Work out the finished part from the listing and answer in its coordinate system (mm). A direction names the side the tool comes from. Give positions to 0.01 mm unless a question says otherwise; leave off trailing zeros. Order: outer loops, then holes, each group sorted by start corner. A loop starts at its lowest first (then second) coordinate and runs counter-clockwise, first axis right, second up. Notation, with made-up numbers: M 50,41.25 L 68,41.25 A22 cw 68,67.25 Z; hole C 2,-31.5 d7. An arc over 180 degrees is marked long. One line per item, written item: value.
from build123d import *

# Parameters (mm, degrees)
SKETCH_R     = 1.6
PAD_DEPTH    = 15
FILLET_R     = 5
SKETCH001_R  = 3
POCKET_DEPTH = 5


with BuildPart() as part:
    # Sketch → Pad (new body)
    with BuildSketch(Plane.XZ):
        with BuildLine():
            ThreePointArc((4.181539, 2.741301), (-4.970119, 0.54582), (3.486952, -3.583457))
            ThreePointArc((3.486952, -56.416543), (15, -30), (3.486952, -3.583457))
            ThreePointArc((3.486952, -56.416543), (-4.970119, -60.54582), (4.181539, -62.741301))
            Line((4.181539, -62.741301), (11.605736, -51.416543))
            ThreePointArc((11.605736, -51.416543), (18, -30), (11.605736, -8.583457))
            Line((4.181539, 2.741301), (11.605736, -8.583457))
        make_face()
        Circle(SKETCH_R, mode=Mode.SUBTRACT)
        with Locations((0, -60)):
            Circle(SKETCH_R, mode=Mode.SUBTRACT)
    extrude(amount=PAD_DEPTH)

    # Fillet
    fillet_edges = [part.edges().sort_by_distance(p)[0] for p in [
        (3.486952, -7.5, -3.583457),
        (3.486952, -7.5, -56.416543),
    ]]
    fillet(fillet_edges, radius=FILLET_R)

    # Sketch001 (on Face5 of Fillet) → Pocket (cut)
    with BuildSketch(Plane.XZ.offset(15)):
        Circle(SKETCH001_R)
        with Locations((0, -60)):
            Circle(SKETCH001_R)
    extrude(amount=-POCKET_DEPTH, mode=Mode.SUBTRACT)


solid = part.part
(1) Section B-B, the plane z = -60 is taken. Give the vertices of the cut face in (x, y).
Findings:
outline: M -5,-15 L -3,-15 L -3,-10 L -1.6,-10 L -1.6,0 L -5,0 Z; M 1.6,-10 L 3,-10 L 3,-15 L 5.98,-15 L 5.98,0 L 1.6,0 Z
(2) Section D-D, the plane z = -46 is taken. Give the vertices of the cut face in (x, y).
Findings:
outline: M 11.26,-15 L 14.57,-15 L 14.57,0 L 11.26,0 Z
(3) Section A-A, the plane x = 0 is taken. Give the vertices of the cut face in (y, z).
Findings:
outline: M -15,-65 L 0,-65 L 0,-61.6 L -10,-61.6 L -10,-63 L -15,-63 Z; M -15,-57 L -10,-57 L -10,-58.4 L 0,-58.4 L 0,-55 L -15,-55 Z; M -15,-5 L 0,-5 L 0,-1.6 L -10,-1.6 L -10,-3 L -15,-3 Z; M -15,3 L -10,3 L -10,1.6 L 0,1.6 L 0,5 L -15,5 Z
(4) Section C-C, the plane y = -2.75 is taken. Give the number of separate pieces and of enclosed holes in the cut face, then the cut area to 3 significant figures.
Findings:
separate pieces: 1
enclosed holes: 2
area: 344 mm^2
(5) Find the intervals of material crossed by probe 1 along Z at (x, y) = (0, -6.5); probe 2 along Z at (x, y) = (0, -13.1); probe 3 along Z at (x, y) = (-4, -1), in increasing order. Write a range as from..to.
Findings:
probe 1: z = -65..-61.6, -58.4..-55, -5..-1.6, 1.6..5
probe 2: z = -65..-63, -57..-55, -5..-3, 3..5
probe 3: z = -63..-57, -3..3
(6) Which of the six approach directions +Z, -Z, +X, -X, +Y, -Y give full straight-line access (tool end or side, diameter ignored) to faces 5 (the flat face through (1.3, -10, -1.3)), 6 (the cylindrical face through (-0.208, -4.93, -58.414))?
Findings:
face 5: -Y
face 6: +Y, -Y
(7) Given P1, Ø3, axis at x = 0, z = 0, coming from the +Y side; P2, Ø5, axis at x = 1.5, z = -6.5, coming from the +Y side; P3, Ø3.5, axis at x = 0, z = -60, coming from the -Y side; P4, Ø4, axis at y = -6.5, z = -12.5, coming from the -X side, each flat-ended and moving along its own axis, determine where each tip first touches the part or whether it passes through.
Findings:
P1: passes through
P2: stops at y = 0
P3: stops at y = -10
P4: stops at x = 9.27
(8) Determine the mould class of faces 1 (the cylindrical face through (-3, -13, 0)), 2 (the cylindrical face through (-1.27, -4.93, -0.97)), 3 (the flat face through (7.84, -7.4, -2.84)), 4 (the flat face through (16, 0, -30)) for opening direction Z: pulls with the +Z half, pulls with the -Z half, needs draft (parallel to the pull), parting line crosses it, or undercut.
Findings:
face 1: undercut
face 2: undercut
face 3: pulls with the +Z half
face 4: needs draft
